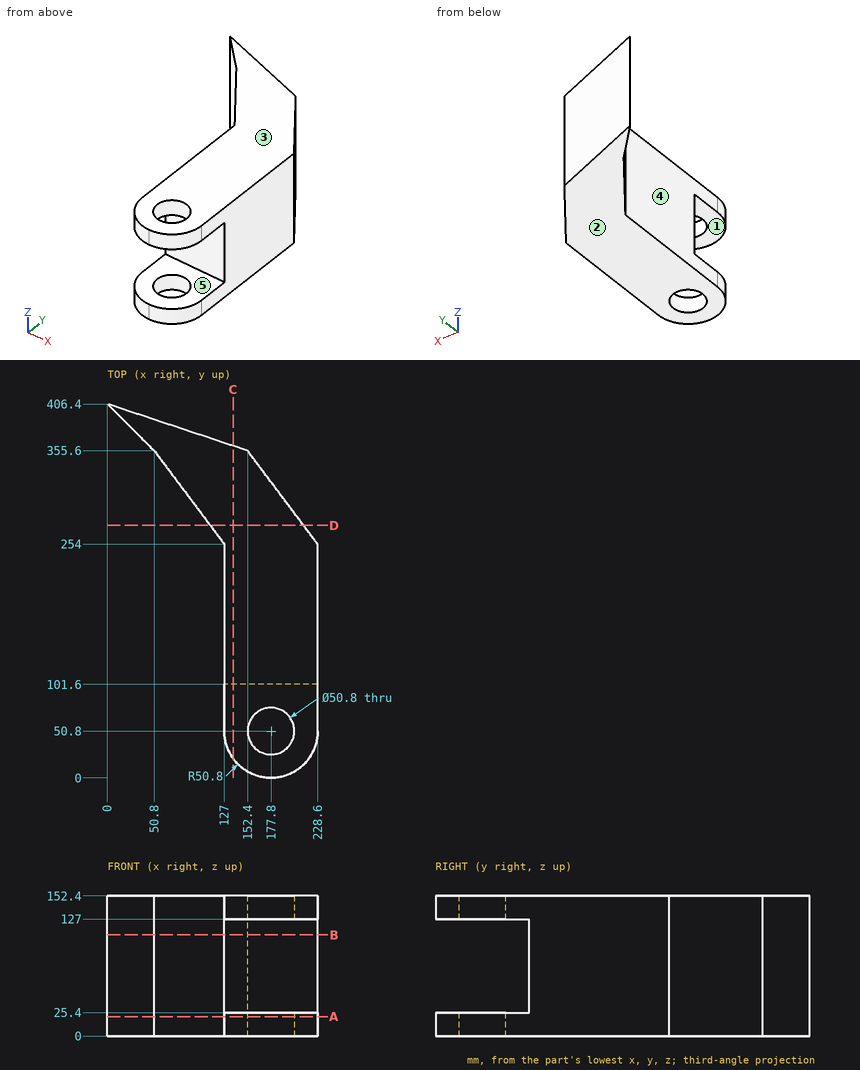
Print and shaded views of the part. All mm, measured from the part's lowest x, y and z. A direction names the side the tool comes from. Give positions to 0.01 mm unless a question says otherwise; leave off trailing zeros. Order: outer loops, then holes, each group sorted by start corner. A loop starts at its lowest first (then second) coordinate and runs counter-clockwise, first axis right, second up. Notation, with made-up numbers: (85, 86.25) - (111, 86.25) arc R12 ccw to (111, 109.25) - close; hole circle Ø11 at (-31.5, 76). An arc over 180 degrees is marked (long way). Use a Markdown table: item, result.
1) 3-axis set-ups, long thin cutter, end or side, ignore diameter. For the marked faces 1 and 2: which of +Z, -Z, +X, -X, +Y, -Y reach the whole face in a straight line?
Checked values:
| item | result |
|---|---|
| face 1 | +X, -X, -Y |
| face 2 | -Z, +X, -X, +Y, -Y |
2) Saw through at A-A on z = 21. List the corners of the cut face in (x, y).
Checked values:
| item | result |
|---|---|
| outline | (0, 406.4) - (50.8, 355.6) - (127, 254) - (127, 50.8) arc R50.8 ccw to (177.8, 0) arc R50.8 ccw to (228.6, 50.8) - (228.6, 254) - (152.4, 355.6) - close; hole circle Ø50.8 at (177.8, 50.8) |
3) Probe L1, parallel to Z at x = 182, y = 89; L2, parallel to X at y = 50, z = 140; L3, parallel to Y at x = 177.8, z = 132.5. List the from-to ranges inside material, lowest first. Write a range as from..to.
Checked values:
| item | result |
|---|---|
| L1 | 0..25.4, 127..152.4 |
| L2 | 127.01..152.41, 203.19..228.59 |
| L3 | 0..25.4, 76.2..321.73 |
4) Flat gauge pins, fed straight in: P1, Ø1, axis at x = 201, z = 82.5, coming from the +Y side; P2, Ø4, axis at x = 62.5, z = 18, coming from the -Y side; P3, Ø12, axis at y = 274, z = 27.5, coming from the -X side. Where does each tip first touch, or does it go through?
Checked values:
| item | result |
|---|---|
| P1 | y = 291.47 |
| P2 | y = 337.33 |
| P3 | x = 107.5 |
5) Saw through at B-B on z = 110. List the corners of the cut face in (x, y), plus the area to 3 significant figures.
Checked values:
| item | result |
|---|---|
| outline | (0, 406.4) - (50.8, 355.6) - (127, 254) - (127, 101.6) - (228.6, 101.6) - (228.6, 254) - (152.4, 355.6) - close |
| area | 28,400 mm² |
6) Saw through at D-D on y = 274.5. List the corners of the cut face in (x, z) (3 decimals), plus the area to 3 significant figures.
Checked values:
| item | result |
|---|---|
| outline | (111.625, 0) - (213.225, 0) - (213.225, 152.4) - (111.625, 152.4) - close |
| area | 15,500 mm² |
7) Saw through at C-C on x = 136.5. List the corners of the cut face in (y, z), plus the area to 3 significant figures.
Checked values:
| item | result |
|---|---|
| outline | (21.22, 0) - (360.9, 0) - (360.9, 152.4) - (21.22, 152.4) - (21.22, 127) - (101.6, 127) - (101.6, 25.4) - (21.22, 25.4) - close |
| area | 43,600 mm² |
8) Two-plate mould, pull along Z, no slides. Class the marked faces 3, 4 and 5: +Z half, -Z half, draft (parallel to the pull), parting line (faces both ways), or undercut.
Checked values:
| item | result |
|---|---|
| face 3 | +Z half |
| face 4 | draft |
| face 5 | undercut |
